Part model, mm, in its own coordinate system. A direction names the side the tool comes from. Give positions to 0.01 mm unless a question says otherwise; leave off trailing zeros. Order: outer loops, then holes, each group sorted by start corner. A loop starts at its lowest first (then second) coordinate and runs counter-clockwise, first axis right, second up. Notation, with made-up numbers: (28, 6) -> (62, 6) arc R33 cw to (62, 43) -> close; hole circle Ø8 at (27, 32.25). An arc over 180 degrees is marked (long way). Write item = value, one per line. Start each with the question number.
(1) Saw through at A-A, the plane x = -53. List the corners of the cut face in (y, z), then the cut area to 3 significant figures.
(2) Saw through at C-C, the plane y = 106.75. List the corners of the cut face in (x, z).
(3) Probe line 1 along X through (y, z) = (106, 26); line 2 along Y through (x, z) = (-110, 26.5); line 3 along Y through (x, z) = (-53, 26). List the from-to ranges inside material, lowest first. Write a range as from..to.
(4) Saw through at B-B, the plane y = 78.5. List the corners of the cut face in (x, z), then the cut area to 3 significant figures.
(5) Flat gauge pins, fed straight in: pin 1 (5 mm diameter, centred on x = -110, y = 106.75, fed in from +Z); pin 2 (2.5 mm diameter, centred on x = -53, y = 13, fed in from +Z); pin 3 (10 mm diameter, centred on y = 57, z = 64.5, fed in from -X); pin 4 (1 mm diameter, centred on y = 87, z = 75, fed in from -X). Where does each tip first touch, or does it go through?
(6) Two-plate mould, pull along X, no slides. Class faces 5 (the cylindrical face through (-18.016, 59.16, 30.007)), 6 (the flat face through (8.89, 59.16, 74.37)), 7 (the cylindrical face through (-40, 7, 27)): pulls with the +X half, pulls with the -X half, needs draft (parallel to the pull), parting line crosses it, or undercut.
(7) Saw through at D-D, the plane x = -100. List the corners of the cut face in (y, z), then the cut area to 3 significant figures.
(8) Which spindle directions (+Z, -Z, +X, -X, +Y, -Y) get a long thin tool onto all of the face, cutting with end or side? Do faces 1 (the flat face through (-0.352, 60.63, 54.438)), 2 (the cylindrical face through (-4.4, 113, 47.4)), 3 (the flat face through (-71, 59, 28.618)), 4 (the cylindrical face through (-40, 113, 27)). Say none if no direction does.
from build123d import *

# Parameters (mm, degrees)
BOSS_EXTRU_1_DEPTH      = 120
ENL_V_MAT_EXTRU_1_DEPTH = 188.009777727
ENL_V_MAT_EXTRU_2_DEPTH = 180.784310366
ESQUISSE6_R             = 2
ENL_V_MAT_EXTRU_3_DEPTH = 188.009777727
ESQUISSE7_R             = 2
ENL_V_MAT_EXTRU_4_DEPTH = 180.784310366
ESQUISSE8_R             = 2
ENL_V_MAT_EXTRU_5_DEPTH = 188.009777727
ESQUISSE9_R             = 2
ENL_V_MAT_EXTRU_6_DEPTH = 180.784310366


with BuildPart() as part:
    # Esquisse3 → Boss.-Extru.1 (new body)
    with BuildSketch(Plane(origin=(0, 0, 0), x_dir=(1, 0, 0), z_dir=(0, 1, 0))):
        with BuildLine():
            ThreePointArc((-25, -28.618176043), (-27.104360033, -26.633694209), (-29.051678093, -24.494897428))
            Line((-29.051678093, -24.494897428), (-115, -24.494897428))
            Line((-115, -24.494897428), (-115, -28.618176043))
            Line((-115, -28.618176043), (-25, -28.618176043))
        make_face()
        with BuildLine():
            ThreePointArc((-10.103808925, -33.509894736), (-18.121448463, -29.943498553), (-25, -24.494897428))
            Line((-25, -24.494897428), (-29.051678093, -24.494897428))
            ThreePointArc((-29.051678093, -24.494897428), (-27.104360033, -26.633694209), (-25, -28.618176043))
            ThreePointArc((-25, -28.618176043), (-19.581111, -32.566548666), (-13.552631037, -35.50107311))
            ThreePointArc((-13.552631037, -35.50107311), (-10.809506446, -36.430132725), (-8.003591765, -37.147577564))
            Line((-8.003591765, -37.147577564), (-10.103808925, -33.509894736))
        make_face()
        with BuildLine():
            Line((35.411933246, -112.345472721), (-8.003591765, -37.147577564))
            ThreePointArc((-8.003591765, -37.147577564), (-10.809506446, -36.430132725), (-13.552631037, -35.50107311))
            Line((-13.552631037, -35.50107311), (31.963111135, -114.336651096))
            Line((31.963111135, -114.336651096), (35.411933246, -112.345472721))
        make_face()
    extrude(amount=BOSS_EXTRU_1_DEPTH)

    # Esquisse4 → Enl_v. mat.-Extru.1 (cut, through all)
    with BuildSketch(Plane.XY.offset(28.618176043)):
        with BuildLine():
            Line((-48, 105), (-48, 15))
            ThreePointArc((-48, 15), (-40, 7), (-32, 15))
            Line((-32, 15), (-32, 105))
            ThreePointArc((-32, 105), (-40, 113), (-48, 105))
        make_face()
    extrude(amount=-ENL_V_MAT_EXTRU_1_DEPTH, mode=Mode.SUBTRACT)

    # Esquisse5 → Enl_v. mat.-Extru.2 (cut, through all)
    with BuildSketch(Plane(origin=(-25.536888865, 0, 14.743729661), x_dir=(0.4999999999999999, 0, 0.8660254037844386), z_dir=(-0.8660254037844387, 0, 0.49999999999999994))):
        with BuildLine():
            Line((46.968515657, 105), (46.968515657, 15))
            ThreePointArc((46.968515657, 15), (38.968515657, 7), (30.968515657, 15))
            Line((30.968515657, 15), (30.968515657, 105))
            ThreePointArc((30.968515657, 105), (38.968515657, 113), (46.968515657, 105))
        make_face()
    extrude(amount=-ENL_V_MAT_EXTRU_2_DEPTH, mode=Mode.SUBTRACT)

    # Esquisse6 → Enl_v. mat.-Extru.3 (cut, through all)
    with BuildSketch(Plane.XY.offset(28.618176043)):
        with Locations((-110, 106.75)):
            Circle(ESQUISSE6_R)
    extrude(amount=-ENL_V_MAT_EXTRU_3_DEPTH, mode=Mode.SUBTRACT)

    # Esquisse7 → Enl_v. mat.-Extru.4 (cut, through all)
    with BuildSketch(Plane(origin=(-25.536888865, 0, 14.743729661), x_dir=(0.4999999999999999, 0, 0.8660254037844386), z_dir=(-0.8660254037844387, 0, 0.49999999999999994))):
        with Locations((110, 106.75)):
            Circle(ESQUISSE7_R)
    extrude(amount=-ENL_V_MAT_EXTRU_4_DEPTH, mode=Mode.SUBTRACT)

    # Esquisse8 → Enl_v. mat.-Extru.5 (cut, through all)
    with BuildSketch(Plane.XY.offset(28.618176043)):
        with Locations((-53, 13)):
            Circle(ESQUISSE8_R)
    extrude(amount=-ENL_V_MAT_EXTRU_5_DEPTH, mode=Mode.SUBTRACT)

    # Esquisse9 → Enl_v. mat.-Extru.6 (cut, through all)
    with BuildSketch(Plane(origin=(-25.536888865, 0, 14.743729661), x_dir=(0.4999999999999999, 0, 0.8660254037844386), z_dir=(-0.8660254037844387, 0, 0.49999999999999994))):
        with Locations((51.968515657, 13)):
            Circle(ESQUISSE9_R)
    extrude(amount=-ENL_V_MAT_EXTRU_6_DEPTH, mode=Mode.SUBTRACT)


solid = part.part
Results list:
q1.outline = (0, 24.49) -> (11, 24.49) -> (11, 28.62) -> (0, 28.62) -> close; (15, 24.49) -> (120, 24.49) -> (120, 28.62) -> (15, 28.62) -> close
q1.area = 478 mm^2
q2.outline = (-115, 24.49) -> (-112, 24.49) -> (-112, 28.62) -> (-115, 28.62) -> close; (-108, 24.49) -> (-47.81, 24.49) -> (-47.81, 28.62) -> (-108, 28.62) -> close; (-32.19, 24.49) -> (-25, 24.49) arc R35 cw to (-10.1, 33.51) -> (-6.51, 39.74) -> (-9.96, 41.73) -> (-13.55, 35.5) arc R38 ccw to (-25, 28.62) -> (-32.19, 28.62) -> close; (-2.15, 55.25) -> (1.3, 53.26) -> (31.91, 106.28) -> (28.46, 108.27) -> close; (30.46, 111.74) -> (33.91, 109.75) -> (35.41, 112.35) -> (31.96, 114.34) -> close
q3.line_1 = -115..-111.85, -108.15..-47.94, -32.06..-23.43
q3.line_2 = 0..104.75, 108.75..120
q3.line_3 = 0..11, 15..120
q4.outline = (-115, 24.49) -> (-48, 24.49) -> (-48, 28.62) -> (-115, 28.62) -> close; (-32, 24.49) -> (-25, 24.49) arc R35 cw to (-10.1, 33.51) -> (-6.6, 39.57) -> (-10.05, 41.56) -> (-13.55, 35.5) arc R38 ccw to (-25, 28.62) -> (-32, 28.62) -> close; (-2.05, 55.42) -> (1.4, 53.43) -> (35.41, 112.35) -> (31.96, 114.34) -> close
q4.area = 650 mm^2
q5.pin_1 = 28.62
q5.pin_2 = through
q5.pin_3 = 0.3
q5.pin_4 = 8.96
q6.face_5 = pulls with the +X half
q6.face_6 = pulls with the -X half
q6.face_7 = undercut
q7.outline = (0, 24.49) -> (120, 24.49) -> (120, 28.62) -> (0, 28.62) -> close
q7.area = 495 mm^2
q8.face_1 = -Z, -X
q8.face_2 = none
q8.face_3 = +Z, -X, +Y, -Y
q8.face_4 = +Z, -Z
